```python
from build123d import *

# Parameters (mm, degrees)
SKETCH_1_W                        = 2000
SKETCH_1_H                        = 262
EXTRUDE_1_DEPTH                   = 200
SKETCH_5_W                        = 232
SKETCH_5_H                        = 238
SKETCH_5_W_2                      = 488
CUT_EXTRUDE_10_DEPTH              = 2027.979032945
SKETCH_7_W                        = 2000
SKETCH_7_H                        = 12
EXTRUDE_13_DEPTH                  = 260
SKETCH_8_R                        = 11
CUT_EXTRUDE_14_DEPTH              = 2027.979032945
PATTERN_LINEAR_3_COUNT            = 16
PATTERN_LINEAR_3_PITCH            = 125
PATTERN_LINEAR_3_COUNT_DIR2       = 2
PATTERN_LINEAR_3_PITCH_DIR2       = 125
SKETCH_10_R                       = 11
CUT_EXTRUDE_16_DEPTH              = 20
PATTERN_LINEAR_5_COUNT            = 2
PATTERN_LINEAR_5_PITCH            = 125
PATTERN_LINEAR_5_COUNT_DIR2       = 2
PATTERN_LINEAR_5_PITCH_DIR2       = 125
CUT_EXTRUDE_START                 = -20
SKETCH_11_R                       = 11
CUT_EXTRUDE_17_DEPTH              = 20
PATTERN_LINEAR_6_COUNT            = 2
PATTERN_LINEAR_6_PITCH            = 125
PATTERN_LINEAR_6_COUNT_DIR2       = 2
PATTERN_LINEAR_6_PITCH_DIR2       = 125
SKETCH_12_R                       = 11
CUT_EXTRUDE_18_DEPTH              = 1550
PATTERN_LINEAR_8_COUNT            = 2
PATTERN_LINEAR_8_PITCH            = 140.2426687
FILLET_1_R                        = 10
FILLET_2_R                        = 10
SKETCH_13_R                       = 11
CUT_EXTRUDE_19_DEPTH              = 2020.871283028
PATTERN_LINEAR_9_COUNT            = 2
PATTERN_LINEAR_9_PITCH            = 125
PATTERN_LINEAR_9_COUNT_DIR2       = 2
PATTERN_LINEAR_9_PITCH_DIR2       = 125
PATTERN_LINEAR_10_COUNT           = 3
PATTERN_LINEAR_10_PITCH           = 500
PATTERN_LINEAR_10_COPY_1_SKETCH_R = 11
PATTERN_LINEAR_10_COPY_1_DEPTH    = 2020.871283028
PATTERN_LINEAR_10_COPY_2_SKETCH_R = 11
PATTERN_LINEAR_10_COPY_2_DEPTH    = 2020.871283028
PATTERN_LINEAR_10_COPY_3_SKETCH_R = 11
PATTERN_LINEAR_10_COPY_3_DEPTH    = 2020.871283028
PATTERN_LINEAR_10_COPY_4_SKETCH_R = 11
PATTERN_LINEAR_10_COPY_4_DEPTH    = 2020.871283028
PATTERN_LINEAR_10_COPY_5_SKETCH_R = 11
PATTERN_LINEAR_10_COPY_5_DEPTH    = 2020.871283028
PATTERN_LINEAR_10_COPY_6_SKETCH_R = 11
PATTERN_LINEAR_10_COPY_6_DEPTH    = 2020.871283028


with BuildPart() as part:
    # 草图1 → 拉伸1 (new body)
    with BuildSketch(Plane.XY):
        with Locations((1000, 131)):
            Rectangle(SKETCH_1_W, SKETCH_1_H)
    extrude(amount=EXTRUDE_1_DEPTH)

    # 草图5 → 拉伸10 (cut, through all)
    with BuildSketch(Plane.XY.offset(200)):
        with Locations((128, 131)):
            Rectangle(SKETCH_5_W, SKETCH_5_H)
        with Locations((500, 131)):
            Rectangle(SKETCH_5_W_2, SKETCH_5_H)
        with Locations((1000, 131)):
            Rectangle(SKETCH_5_W_2, SKETCH_5_H)
        with Locations((1500, 131)):
            Rectangle(SKETCH_5_W_2, SKETCH_5_H)
        with Locations((1872, 131)):
            Rectangle(SKETCH_5_W, SKETCH_5_H)
    extrude(amount=-CUT_EXTRUDE_10_DEPTH, mode=Mode.SUBTRACT)

    # 草图7 → 拉伸13 (add)
    with BuildSketch(Plane.XZ):
        with Locations((1000, 100)):
            Rectangle(SKETCH_7_W, SKETCH_7_H)
    extrude(amount=-EXTRUDE_13_DEPTH)

    # 草图8 → 拉伸14 (cut, through all)
    with BuildSketch(Plane.XZ):
        with Locations(Location((62.5, 37.5, 0), (0, 0, 270))):
            Circle(SKETCH_8_R)
    cut_extrude_14 = extrude(amount=-CUT_EXTRUDE_14_DEPTH, mode=Mode.SUBTRACT)

    # 阵列(线性)3: Cut-Extrude 14 16 × 2
    with Locations(*[(i * PATTERN_LINEAR_3_PITCH, 0, j * PATTERN_LINEAR_3_PITCH_DIR2) for i in range(PATTERN_LINEAR_3_COUNT) for j in range(PATTERN_LINEAR_3_COUNT_DIR2) if (i, j) != (0, 0)]):
        add(cut_extrude_14, mode=Mode.SUBTRACT)

    # 草图10 → 拉伸16 (cut)
    with BuildSketch(Plane.ZY):
        with Locations((37.5, 68.5)):
            Circle(SKETCH_10_R)
    cut_extrude_16 = extrude(amount=-CUT_EXTRUDE_16_DEPTH, mode=Mode.SUBTRACT)

    # 阵列(线性)5: Cut-Extrude 16 2 × 2
    with Locations(*[(0, j * PATTERN_LINEAR_5_PITCH_DIR2, i * PATTERN_LINEAR_5_PITCH) for i in range(PATTERN_LINEAR_5_COUNT) for j in range(PATTERN_LINEAR_5_COUNT_DIR2) if (i, j) != (0, 0)]):
        add(cut_extrude_16, mode=Mode.SUBTRACT)

    # 草图11 → 拉伸17 (cut)
    with BuildSketch(Plane(origin=(2000, 0, 0), x_dir=(0, 0, -1), z_dir=(1, 0, 0)).offset(CUT_EXTRUDE_START)):
        with Locations(Location((-162.5, 68.5, 0), (0, 0, 180))):
            Circle(SKETCH_11_R)
    cut_extrude_17 = extrude(amount=CUT_EXTRUDE_17_DEPTH, mode=Mode.SUBTRACT)

    # 阵列(线性)6: Cut-Extrude 17 2 × 2
    with Locations(*[(0, j * PATTERN_LINEAR_6_PITCH_DIR2, -i * PATTERN_LINEAR_6_PITCH) for i in range(PATTERN_LINEAR_6_COUNT) for j in range(PATTERN_LINEAR_6_COUNT_DIR2) if (i, j) != (0, 0)]):
        add(cut_extrude_17, mode=Mode.SUBTRACT)

    # 草图12 → 拉伸18 (cut)
    with BuildSketch(Plane(origin=(1756, 0, 0), x_dir=(0, 0, -1), z_dir=(1, 0, 0))):
        with Locations((-170.12133435, 131)):
            Circle(SKETCH_12_R)
    cut_extrude_18 = extrude(amount=-CUT_EXTRUDE_18_DEPTH, mode=Mode.SUBTRACT)

    # 阵列(线性)8: 拉伸18 ×2
    with Locations(*[(0, 0, -i * PATTERN_LINEAR_8_PITCH) for i in range(1, PATTERN_LINEAR_8_COUNT)]):
        add(cut_extrude_18, mode=Mode.SUBTRACT)

    # 圆角1
    fillet_1_edges = [part.edges().sort_by_distance(p)[0] for p in [
        (0, 131, 200),
        (0, 131, 0),
        (0, 262, 100),
        (0, 0, 100),
    ]]
    fillet(fillet_1_edges, radius=FILLET_1_R)

    # 圆角2
    fillet_2_edges = [part.edges().sort_by_distance(p)[0] for p in [
        (2000, 131, 200),
        (2000, 131, 0),
        (2000, 262, 100),
        (2000, 0, 100),
    ]]
    fillet(fillet_2_edges, radius=FILLET_2_R)

    # 草图13 → 拉伸19 (cut, through all)
    with BuildSketch(Plane.XY.offset(106)):
        with Locations((437.5, 68.5)):
            Circle(SKETCH_13_R)
    cut_extrude_19 = extrude(amount=-CUT_EXTRUDE_19_DEPTH, mode=Mode.SUBTRACT)

    # 阵列(线性)9: Cut-Extrude 19 2 × 2
    with Locations(*[(i * PATTERN_LINEAR_9_PITCH, j * PATTERN_LINEAR_9_PITCH_DIR2, 0) for i in range(PATTERN_LINEAR_9_COUNT) for j in range(PATTERN_LINEAR_9_COUNT_DIR2) if (i, j) != (0, 0)]):
        add(cut_extrude_19, mode=Mode.SUBTRACT)

    # 阵列(线性)10: 拉伸19 ×3
    with Locations(*[(i * PATTERN_LINEAR_10_PITCH, 0, 0) for i in range(1, PATTERN_LINEAR_10_COUNT)]):
        add(cut_extrude_19, mode=Mode.SUBTRACT)

    # 阵列(线性)10 copy 1 sketch → 阵列(线性)10 copy 1 (cut, through all)
    with BuildSketch(Plane(origin=(500, 125, 106), x_dir=(1, 0, 0), z_dir=(0, 0, 1))):
        with Locations((437.5, 68.5)):
            Circle(PATTERN_LINEAR_10_COPY_1_SKETCH_R)
    extrude(amount=-PATTERN_LINEAR_10_COPY_1_DEPTH, mode=Mode.SUBTRACT)

    # 阵列(线性)10 copy 2 sketch → 阵列(线性)10 copy 2 (cut, through all)
    with BuildSketch(Plane(origin=(1000, 125, 106), x_dir=(1, 0, 0), z_dir=(0, 0, 1))):
        with Locations((437.5, 68.5)):
            Circle(PATTERN_LINEAR_10_COPY_2_SKETCH_R)
    extrude(amount=-PATTERN_LINEAR_10_COPY_2_DEPTH, mode=Mode.SUBTRACT)

    # 阵列(线性)10 copy 3 sketch → 阵列(线性)10 copy 3 (cut, through all)
    with BuildSketch(Plane(origin=(625, 0, 106), x_dir=(1, 0, 0), z_dir=(0, 0, 1))):
        with Locations((437.5, 68.5)):
            Circle(PATTERN_LINEAR_10_COPY_3_SKETCH_R)
    extrude(amount=-PATTERN_LINEAR_10_COPY_3_DEPTH, mode=Mode.SUBTRACT)

    # 阵列(线性)10 copy 4 sketch → 阵列(线性)10 copy 4 (cut, through all)
    with BuildSketch(Plane(origin=(1125, 0, 106), x_dir=(1, 0, 0), z_dir=(0, 0, 1))):
        with Locations((437.5, 68.5)):
            Circle(PATTERN_LINEAR_10_COPY_4_SKETCH_R)
    extrude(amount=-PATTERN_LINEAR_10_COPY_4_DEPTH, mode=Mode.SUBTRACT)

    # 阵列(线性)10 copy 5 sketch → 阵列(线性)10 copy 5 (cut, through all)
    with BuildSketch(Plane(origin=(625, 125, 106), x_dir=(1, 0, 0), z_dir=(0, 0, 1))):
        with Locations((437.5, 68.5)):
            Circle(PATTERN_LINEAR_10_COPY_5_SKETCH_R)
    extrude(amount=-PATTERN_LINEAR_10_COPY_5_DEPTH, mode=Mode.SUBTRACT)

    # 阵列(线性)10 copy 6 sketch → 阵列(线性)10 copy 6 (cut, through all)
    with BuildSketch(Plane(origin=(1125, 125, 106), x_dir=(1, 0, 0), z_dir=(0, 0, 1))):
        with Locations((437.5, 68.5)):
            Circle(PATTERN_LINEAR_10_COPY_6_SKETCH_R)
    extrude(amount=-PATTERN_LINEAR_10_COPY_6_DEPTH, mode=Mode.SUBTRACT)


solid = part.part
```
Geometry: final body of the model. Coordinates: model frame, mm. A direction names the side the tool comes from. Round coordinates to 2 decimals unless told otherwise and drop trailing zeros. Order: outer loops, then holes, each group sorted by start corner. A loop starts at its lowest first (then second) coordinate and runs counter-clockwise, first axis right, second up. Notation, with made-up numbers: (-33, 14.25) -> (23, 14.25) arc R25 ccw to (23, 27.25) -> close; hole circle Ø11 at (87.25, 70). An arc over 180 degrees is marked (long way). Use one line per item in the form item = value. Start each with the question number.
1. Reachability of faces 1 (the face through (2000, 129, 99)), 2 (the face through (1497, 129, 106)), 3 (the face through (1497, 129, 94)) from +Z, -Z, +X, -X, +Y, -Y: full face, straight path, thin tool, end or side. Return the list, or none.
2. Pin query (flat end, axial travel): pin 1 Ø13 at (x, z) = (937.5, 162.5) entering from -Y; pin 2 Ø1.5 at (x, y) = (1129.5, 32.5) entering from +Z. Return the tip coordinate at first contact, or that it passes through.
3. Cut plane A-A (x = 723.5). Return the cut outline in (y, z).
4. Draft query along Y for faces 4 (the face through (995, 5, 200)), 5 (the face through (997, 250, 48)). Return one class per face: pulls with the +Y half, pulls with the -Y half, needs draft (parallel to the pull), parting line crosses it, or undercut.
5. Line query: probe 1 along X at (y, z) = (148, 38.5); probe 2 along Y at (x, z) = (1062.5, 100); probe 3 along Z at (x, y) = (562.5, 3.5). Output: solid intervals per line, ascending.
Solution:
q1.face_1 = +Z, -Z, +X, +Y, -Y
q1.face_2 = +Z
q1.face_3 = -Z
q2.pin_1 = through
q2.pin_2 = 106
q3.outline = (0, 0) -> (12, 0) -> (12, 94) -> (250, 94) -> (250, 0) -> (262, 0) -> (262, 200) -> (250, 200) -> (250, 106) -> (12, 106) -> (12, 200) -> (0, 200) -> close
q4.face_4 = needs draft
q4.face_5 = undercut
q5.probe_1 = 0 to 12, 244 to 256, 744 to 756, 1244 to 1256, 1744 to 1756, 1988 to 2000
q5.probe_2 = 0 to 57.5, 79.5 to 182.5, 204.5 to 262
q5.probe_3 = 0 to 26.5, 48.5 to 151.5, 173.5 to 200
